Answer from the drawing. Dimensions are ordinates in mm from the lowest x, y and z of the part. Round coordinates to 2 decimals unless told otherwise and drop trailing zeros. Order: outer loops, then holes, each group sorted by start corner. A loop starts at its lowest first (then second) coordinate and runs counter-clockwise, first axis right, second up. Notation, with made-up numbers: (37.5, 73.5) -> (66.5, 73.5) arc R26 cw to (66.5, 91.5) -> close; hole circle Ø4 at (-27.75, 79). An arc over 180 degrees is marked (long way). Use a Markdown table: item, result. Add a question column.
Item 1: A cutting plane is placed at D-D, the plane z = 40.5. Determine the outline of the cut face in (x, y).
Item 2: A cutting plane is placed at A-A, the plane x = 119.5. Determine the outline of the cut face in (y, z).
Item 3: A flat-ended cylindrical pin translates along its axis: P1, Ø0.9, axis at y = 2, z = 40, coming from the -X side. Find the tip coordinate at first contact, or state that the pin passes through.
Item 4: Find the intervals of material crossed by L1, parallel to Z at x = 103.75, y = 1; L2, parallel to X at y = 0.8, z = 7; L3, parallel to X at y = 0.55, z = 68.5, in increasing order. Write a range as [from, to].
Item 5: A cutting plane is placed at B-B, the plane y = 1.75. Give the number of separate pieces and of enclosed holes in the cut face, plus the area to 3 significant figures.
Item 6: A cutting plane is placed at C-C, the plane z = 7. Determine the outline of the cut face in (x, y).
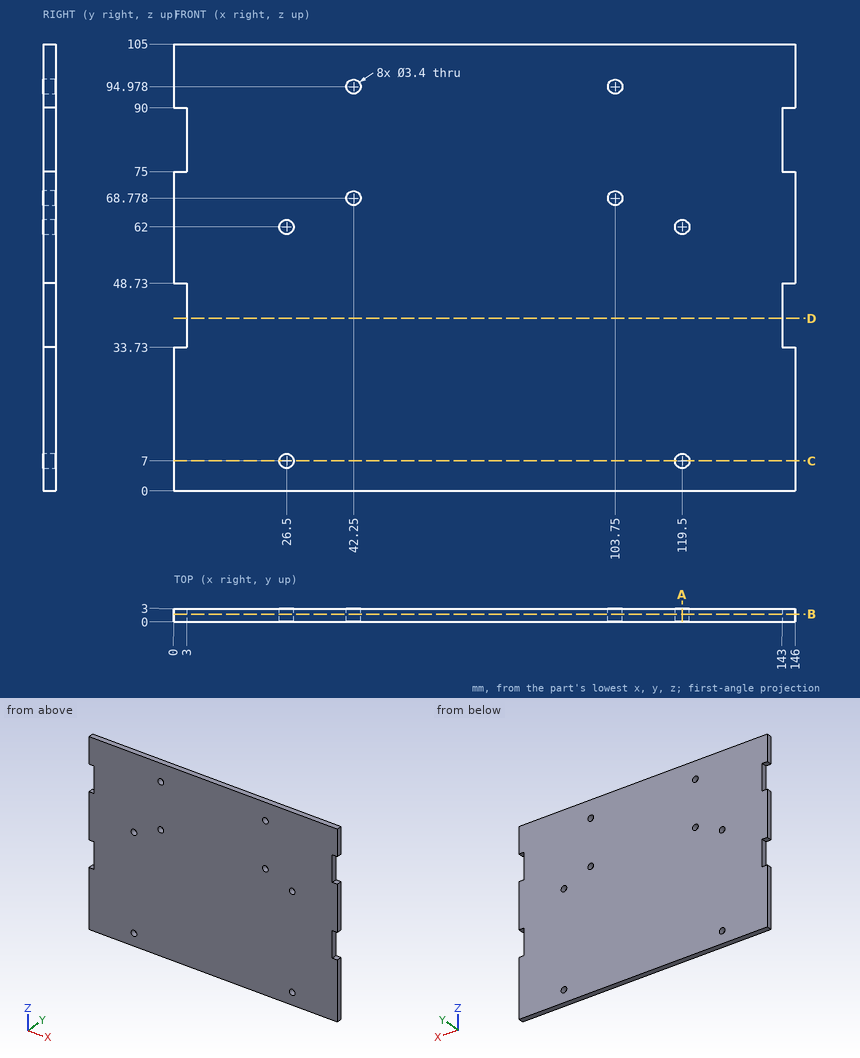
Reported:
| question | item | result |
|---|---|---|
| 1 | outline | (3, 0) -> (143, 0) -> (143, 3) -> (3, 3) -> close |
| 2 | outline | (0, 0) -> (3, 0) -> (3, 5.3) -> (0, 5.3) -> close; (0, 8.7) -> (3, 8.7) -> (3, 60.3) -> (0, 60.3) -> close; (0, 63.7) -> (3, 63.7) -> (3, 105) -> (0, 105) -> close |
| 3 | P1 | x = 3 |
| 4 | L1 | [0, 67.08], [70.48, 93.28], [96.68, 105] |
| 4 | L2 | [0, 24.8], [28.2, 117.8], [121.2, 146] |
| 4 | L3 | [0, 40.57], [43.93, 102.07], [105.43, 146] |
| 5 | separate pieces | 1 |
| 5 | enclosed holes | 8 |
| 5 | area | 15,100 mm² |
| 6 | outline | (0, 0) -> (24.8, 0) -> (24.8, 3) -> (0, 3) -> close; (28.2, 0) -> (117.8, 0) -> (117.8, 3) -> (28.2, 3) -> close; (121.2, 0) -> (146, 0) -> (146, 3) -> (121.2, 3) -> close |
